```python
from build123d import *

# Parameters (mm, degrees)
SKETCH_1_W      = 22
SKETCH_1_H      = 22
SKETCH_1_R      = 1.55
EXTRUDE_1_DEPTH = 5
EXTRUDE_2_DEPTH = 127


with BuildPart() as part:
    # 草图1 → 凸台-拉伸1 (new body)
    with BuildSketch(Plane(origin=(0, 0, 0), x_dir=(1, 0, 0), z_dir=(0, 1, 0))):
        Rectangle(SKETCH_1_W, SKETCH_1_H)
        with Locations(Location((-7.424621202, 7.424621202, 0), (0, 0, 270))):
            Circle(SKETCH_1_R, mode=Mode.SUBTRACT)
        with Locations(Location((7.424621202, 7.424621202, 0), (0, 0, 270))):
            Circle(SKETCH_1_R, mode=Mode.SUBTRACT)
        with Locations(Location((7.424621202, -7.424621202, 0), (0, 0, 270))):
            Circle(SKETCH_1_R, mode=Mode.SUBTRACT)
        with Locations(Location((-7.424621202, -7.424621202, 0), (0, 0, 270))):
            Circle(SKETCH_1_R, mode=Mode.SUBTRACT)
    extrude(amount=EXTRUDE_1_DEPTH)

    # 草图2 → 凸台-拉伸2 (add)
    with BuildSketch(Plane(origin=(0, 5, 0), x_dir=(1, 0, 0), z_dir=(0, 1, 0))):
        Polygon((0, 6), (-6, 0), (0, -6), (6, 0), align=None)
    extrude(amount=EXTRUDE_2_DEPTH)


solid = part.part
```
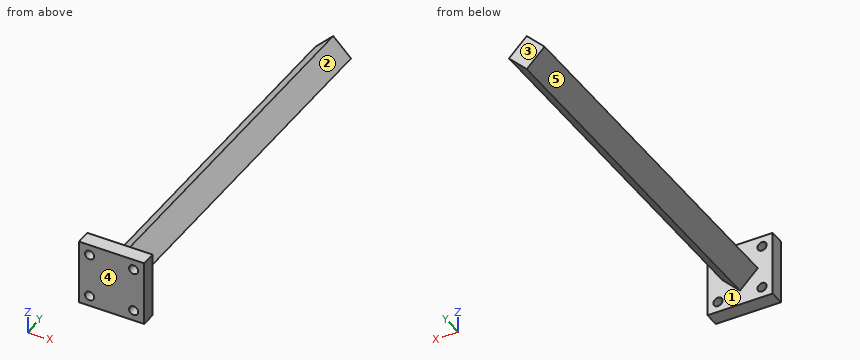
Source: CAD feature listing. Evaluate the final solid. Frame: model axes, mm. Face numbers are marked on the shaded views. A direction names the side the tool comes from. Give positions to 0.01 mm unless a question says otherwise; leave off trailing zeros. Loops run counter-clockwise (first coordinate to the right, second up) from the corner with the lowest first, then second, coordinate; pieces in that order, holes last. Notation, with made-up numbers: (47, 73.5) -> (61, 73.5) arc R16 cw to (61, 101.5) -> close; hole circle Ø6 at (47.5, -3.5). An arc over 180 degrees is marked (long way). Put each result on its own line as item: value. Start each with the question number.
1) Cut plane A-A (x = 1.75). Return loops of the section in (y, z).
2) Material intervals for probe 1 along Y at (x, z) = (5.75, -5.5); probe 2 along X at (y, z) = (66, 2.5); probe 3 along Z at (x, y) = (-4, 90.5), sorted ascending.
3) Cut plane B-B (z = 3.25). Return loops of the section in (x, y), then the cut area to 4 significant figures.
4) Reachability of the marked faces 1, 2, 3, 4 and 5 from +Z, -Z, +X, -X, +Y, -Y: full face, straight path, thin tool, end or side. Return the list, or none.
5) Contact query for flat-ended pins moving along their axis: P1, Ø1.5, axis at y = 115.5, z = 6, coming from the -X side; P2, Ø3.5, axis at x = -7.42, z = 7.42, coming from the +Y side; P3, Ø2, axis at y = 73, z = 6, coming from the +X side; P4, Ø2, axis at y = 77, z = -7.5, coming from the -X side. Output: stop coordinate, or through.
6) Cut plane C-C (y = 19). Return loops of the section in (x, z).
Results are:
1. outline: (0, -11) -> (5, -11) -> (5, -4.25) -> (132, -4.25) -> (132, 4.25) -> (5, 4.25) -> (5, 11) -> (0, 11) -> close
2. probe 1: y = 0 to 5
2. probe 2: x = -3.5 to 3.5
2. probe 3: z = -2 to 2
3. outline: (-11, 0) -> (11, 0) -> (11, 5) -> (2.75, 5) -> (2.75, 132) -> (-2.75, 132) -> (-2.75, 5) -> (-11, 5) -> close
3. area: 808.5 mm2
4. face 1: +Y
4. face 2: +Z, +X, +Y
4. face 3: +Z, -Z, +X, -X, +Y
4. face 4: +Z, -Z, +X, -X, -Y
4. face 5: -Z, -X, +Y
5. P1: stops at x = -0.75
5. P2: stops at y = 5
5. P3: stops at x = 1
5. P4: passes through
6. outline: (-6, 0) -> (0, -6) -> (6, 0) -> (0, 6) -> close
